Can you work these out from the model? Positions are in its coordinate system, mm. Face numbers are marked on the shaded views. A direction names the side the tool comes from. Round coordinates to 2 decimals unless told otherwise and drop trailing zeros. Loops run counter-clockwise (first coordinate to the right, second up) from the corner with the lowest first, then second, coordinate; pieces in that order, holes last.
from build123d import *

# Parameters (mm, degrees)
F2_R     = 40
F2_R_2   = 32.5
F3_DEPTH = 3
F4_W     = 8
F4_H     = 10
F6_R     = 5
F7_DEPTH = 102.001
F8_R     = 2


with BuildPart() as f1:
    # F0 (on Front) → F1 (revolve)
    with BuildSketch(Plane.XZ):
        Polygon((0, 38), (0, 0), (22.5, 0), (22.5, 5), (10, 5), (10, 18), (15, 18), (15, 22), (12, 22), (12, 28), (6, 38), align=None)
    revolve(axis=Axis((0, 0, 28.7462979999), (0, 0, 1)))

    # F2 (on Front) → F3 (join, symmetric)
    with BuildSketch(Plane.XZ):
        with Locations((0, 60)):
            Circle(F2_R)
        with Locations((0, 63)):
            Circle(F2_R_2, mode=Mode.SUBTRACT)
    extrude(amount=F3_DEPTH, both=True)

    # F4 (on Front) → F5 (revolve)
    with BuildSketch(Plane.XZ):
        with Locations((4, 97)):
            Rectangle(F4_W, F4_H)
    revolve(axis=Axis((0, 0, 94.4946174344), (0, 0, -1)))

    # F6 (on face) → F7 (cut, through all)
    with BuildSketch(Plane.XY.offset(102)):
        Circle(F6_R)
    extrude(amount=-F7_DEPTH, mode=Mode.SUBTRACT)

    # F8
    f8_edges = [f1.edges().sort_by_distance(p)[0] for p in [
        (-8, 0, 102),
    ]]
    fillet(f8_edges, radius=F8_R)


solid = f1.part
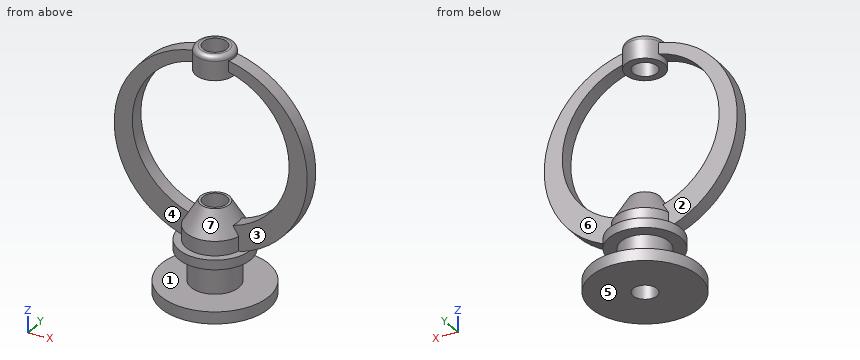
(1) If we section it at A-A, the plane x = 0: State how many separate pieces and enclosed holes the cut face has, then the cut area to 3 significant figures.
Worked answers:
separate pieces: 4
enclosed holes: 0
area: 607 mm2
(2) If I drill on line 1 (X direction, y = -1.5, z = 33); line 2 (Y direction, x = 0, z = 99.75); line 3 (Y direction, x = 0, z = 21), over which ranges is the centre line in solid material (lowest first)?
Worked answers:
line 1: x = -29.51 to -12.5, -8.87 to -4.77, 4.77 to 8.87, 12.5 to 29.51
line 2: y = -8 to -5, 5 to 8
line 3: y = -15 to -5, 5 to 15
(3) If we mould it in two halves opening along Z, with no side actions, what happens to the marked faces 5, 6 and 7? For each: released by +Z, released by -Z, zero draft, split by the parting line, or undercut.
Worked answers:
face 5: released by -Z
face 6: zero draft
face 7: undercut
(4) For the marked faces 1, 2, 3 and 4, which set-ups out of +Z, -Z, +X, -X, +Y, -Y let a thin tool reach every point of the face, with its end or its side?
Worked answers:
face 1: none
face 2: +Z, -X, +Y
face 3: +Z, +X, -Y
face 4: +Z, -X, -Y
(5) If we section it at B-B, the plane z = 81.5: List the corners of the cut face in (x, y) for me, then the cut area to 3 significant figures.
Worked answers:
outline: (-33.73, -3) - (-26.72, -3) - (-26.72, 3) - (-33.73, 3) - close; (26.72, -3) - (33.73, -3) - (33.73, 3) - (26.72, 3) - close
area: 84.1 mm2
(6) Will these pins go through, and if not, where does the flat tip stop? P1, Ø8, axis at x = 14, y = -7.5, coming from the +Z side; P2, Ø8, axis at x = 8.5, z = 91, coming from the -Y side; P3, Ø8, axis at x = 0, y = 0, coming from the +Z side; P4, Ø12, axis at x = -10, y = 16, coming from the +Z side.
Worked answers:
P1: stops at z = 28.2
P2: stops at y = -6.53
P3: passes through
P4: stops at z = 22
(7) If we section it at D-D, the plane z = 10.5: List the corners of the cut face in (x, y) for me.
Worked answers:
outline: circle Ø20 at (0, 0); hole circle Ø10 at (0, 0)
(8) If we section it at C-C, the plane x = -31: List the corners of the cut face in (y, z) for me.
Worked answers:
outline: (-3, 34.72) - (3, 34.72) - (3, 53.24) - (-3, 53.24) - close; (-3, 72.76) - (3, 72.76) - (3, 85.28) - (-3, 85.28) - close
